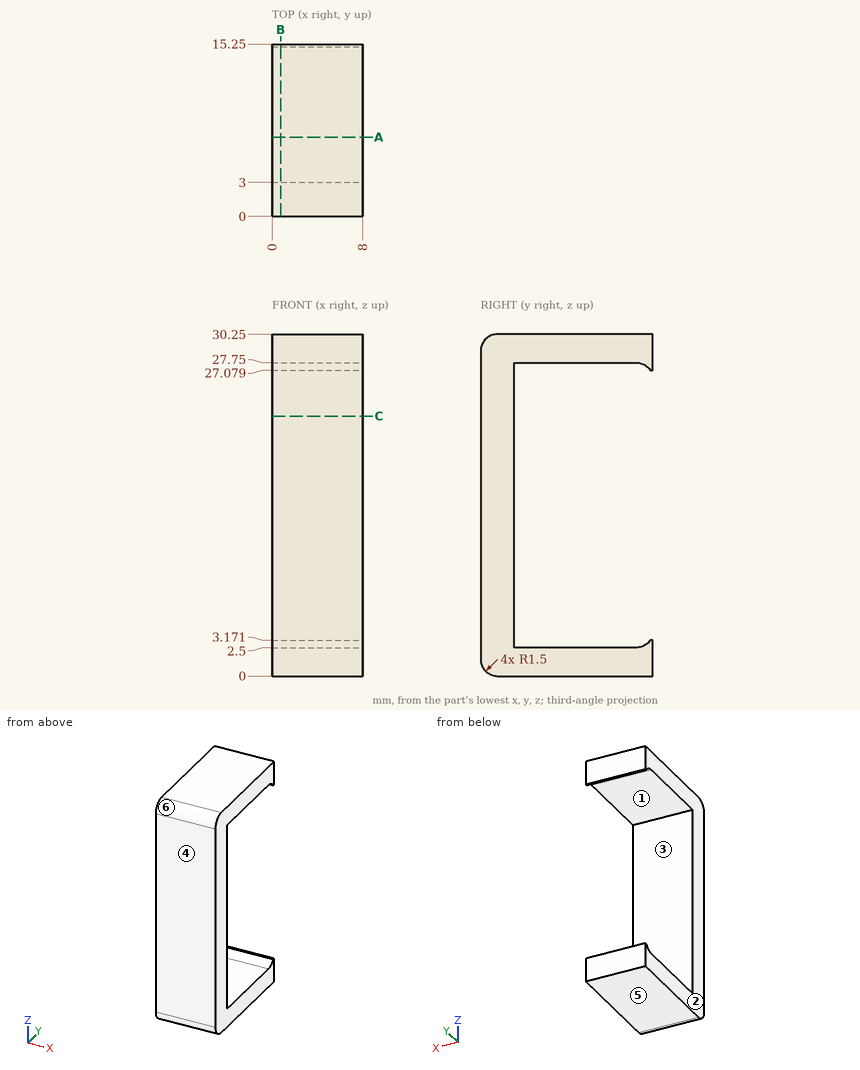
Verification items for this drawing (mm, ordinates from the low corner). A direction names the side the tool comes from. Coordinates: 2 decimals unless noted, no trailing zeros. Loops run counter-clockwise (first coordinate to the right, second up) from the corner with the lowest first, then second, coordinate; pieces in that order, holes last. Notation, with made-up numbers: (-37.75, 4.25) - (20.25, 4.25) arc R20 cw to (20.25, 20.25) - close; hole circle Ø4 at (-6, 85). An arc over 180 degrees is marked (long way). One line per item, written item: value. Start each with the question number.
(1) Mould release check, pull along Z, two halves, no side actions. Record for the marked faces 3, 4, 5 and 6: released by +Z, released by -Z, zero draft, split by the parting line, or undercut.
(2) Cross-section at A-A on y = 7. Enter the section's corners in (x, z), plus the area to 3 significant figures.
(3) Cross-section at B-B on x = 0.75. Enter the section's corners in (y, z), plus the area to 3 significant figures.
(4) Tool access check on the marked faces 1 and 2. Record the directions out of +Z, -Z, +X, -X, +Y, -Y that give a thin tool (end or side, any length) a straight path to the whole face; none if there is none.
(5) Material ranges on line 1 (Z direction, x = 3.25, y = 9.5); line 2 (Y direction, x = 2.25, z = 6); line 3 (Y direction, x = 2, z = 27.5), recorded low to high. Write a range as [from, to].
(6) Cross-section at C-C on z = 23. Enter the section's corners in (x, y), plus the area to 3 significant figures.
Results below:
1. face 3: undercut
1. face 4: zero draft
1. face 5: released by -Z
1. face 6: released by +Z
2. outline: (0, 0) - (8, 0) - (8, 2.5) - (0, 2.5) - close; (0, 27.75) - (8, 27.75) - (8, 30.25) - (0, 30.25) - close
2. area: 40.0 mm2
3. outline: (0, 1.5) arc R1.5 ccw to (1.5, 0) - (15.25, 0) - (15.25, 3.17) - (15, 3.17) arc R1.5 cw to (13.75, 2.5) - (3, 2.5) - (3, 27.75) - (13.75, 27.75) arc R1.5 cw to (15, 27.08) - (15.25, 27.08) - (15.25, 30.25) - (1.5, 30.25) arc R1.5 ccw to (0, 28.75) - close
3. area: 152 mm2
4. face 1: +X, -X
4. face 2: +Z, -Z, -X, +Y, -Y
5. line 1: z = [0, 2.5], [27.75, 30.25]
5. line 2: y = [0, 3]
5. line 3: y = [0, 3], [14.58, 15.25]
6. outline: (0, 0) - (8, 0) - (8, 3) - (0, 3) - close
6. area: 24.0 mm2
